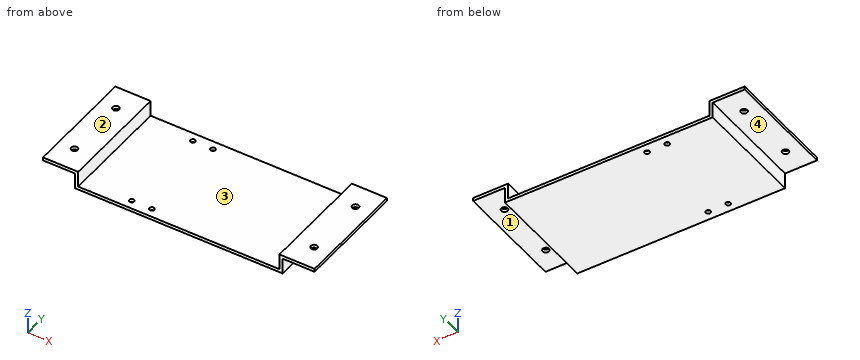
```python
from build123d import *

# Parameters (mm, degrees)
SKETCH1_W           = 126
SKETCH1_H           = 70
BOSS_EXTRUDE1_DEPTH = 2
CUT_EXTRUDE1_REACH  = 4
SKETCH2_R           = 1.5
BOSS_EXTRUDE2_DEPTH = 70
CUT_EXTRUDE2_REACH  = 4
SKETCH4_R           = 2


with BuildPart() as part:
    # Sketch1 → Boss-Extrude1 (new body)
    with BuildSketch(Plane.XY):
        Rectangle(SKETCH1_W, SKETCH1_H)
    extrude(amount=BOSS_EXTRUDE1_DEPTH)

    # Sketch2 → Cut-Extrude1 (cut, up to next)
    with BuildSketch(Plane.XY.offset(2), mode=Mode.PRIVATE) as cut_extrude1_sk1:
        with Locations((-20.4, 29.5)):
            Circle(SKETCH2_R)
    cut_extrude1_tool1 = extrude(cut_extrude1_sk1.sketch, amount=-CUT_EXTRUDE1_REACH, mode=Mode.PRIVATE) & part.part
    add(cut_extrude1_tool1.solids().sort_by_distance((-20.4, 29.5, 2))[0], mode=Mode.SUBTRACT)
    # Sketch2 → Cut-Extrude1 (cut, up to next)
    with BuildSketch(Plane.XY.offset(2), mode=Mode.PRIVATE) as cut_extrude1_sk2:
        with Locations((-33, 29.5)):
            Circle(SKETCH2_R)
    cut_extrude1_tool2 = extrude(cut_extrude1_sk2.sketch, amount=-CUT_EXTRUDE1_REACH, mode=Mode.PRIVATE) & part.part
    add(cut_extrude1_tool2.solids().sort_by_distance((-33, 29.5, 2))[0], mode=Mode.SUBTRACT)
    # Sketch2 → Cut-Extrude1 (cut, up to next)
    with BuildSketch(Plane.XY.offset(2), mode=Mode.PRIVATE) as cut_extrude1_sk3:
        with Locations((-20.4, -29.5)):
            Circle(SKETCH2_R)
    cut_extrude1_tool3 = extrude(cut_extrude1_sk3.sketch, amount=-CUT_EXTRUDE1_REACH, mode=Mode.PRIVATE) & part.part
    add(cut_extrude1_tool3.solids().sort_by_distance((-20.4, -29.5, 2))[0], mode=Mode.SUBTRACT)
    # Sketch2 → Cut-Extrude1 (cut, up to next)
    with BuildSketch(Plane.XY.offset(2), mode=Mode.PRIVATE) as cut_extrude1_sk4:
        with Locations((-33, -29.5)):
            Circle(SKETCH2_R)
    cut_extrude1_tool4 = extrude(cut_extrude1_sk4.sketch, amount=-CUT_EXTRUDE1_REACH, mode=Mode.PRIVATE) & part.part
    add(cut_extrude1_tool4.solids().sort_by_distance((-33, -29.5, 2))[0], mode=Mode.SUBTRACT)

    # Sketch3 → Boss-Extrude2 (add)
    with BuildSketch(Plane(origin=(0, 35, 0), x_dir=(1, 0, 0), z_dir=(0, 1, 0))):
        Polygon((-63, 0), (-63, -12), (-85, -12), (-85, -10), (-65, -10), (-65, 0), align=None)
    boss_extrude2 = extrude(amount=-BOSS_EXTRUDE2_DEPTH)

    # Mirror1: Boss-Extrude2 across plane
    add(boss_extrude2.mirror(Plane(origin=(0, 0, 0), x_dir=(0, 0, 1), z_dir=(1, 0, 0))))

    # Sketch4 → Cut-Extrude2 (cut, up to next)
    with BuildSketch(Plane(origin=(0, 0, 10), x_dir=(-1, 0, 0), z_dir=(0, 0, -1)), mode=Mode.PRIVATE) as cut_extrude2_sk1:
        with Locations((-75, 20)):
            Circle(SKETCH4_R)
    cut_extrude2_tool1 = extrude(cut_extrude2_sk1.sketch, amount=-CUT_EXTRUDE2_REACH, mode=Mode.PRIVATE) & part.part
    add(cut_extrude2_tool1.solids().sort_by_distance((75, 20, 10))[0], mode=Mode.SUBTRACT)
    # Sketch4 → Cut-Extrude2 (cut, up to next)
    with BuildSketch(Plane(origin=(0, 0, 10), x_dir=(-1, 0, 0), z_dir=(0, 0, -1)), mode=Mode.PRIVATE) as cut_extrude2_sk2:
        with Locations((-75, -20)):
            Circle(SKETCH4_R)
    cut_extrude2_tool2 = extrude(cut_extrude2_sk2.sketch, amount=-CUT_EXTRUDE2_REACH, mode=Mode.PRIVATE) & part.part
    add(cut_extrude2_tool2.solids().sort_by_distance((75, -20, 10))[0], mode=Mode.SUBTRACT)
    # Sketch4 → Cut-Extrude2 (cut, up to next)
    with BuildSketch(Plane(origin=(0, 0, 10), x_dir=(-1, 0, 0), z_dir=(0, 0, -1)), mode=Mode.PRIVATE) as cut_extrude2_sk3:
        with Locations((75, 20)):
            Circle(SKETCH4_R)
    cut_extrude2_tool3 = extrude(cut_extrude2_sk3.sketch, amount=-CUT_EXTRUDE2_REACH, mode=Mode.PRIVATE) & part.part
    add(cut_extrude2_tool3.solids().sort_by_distance((-75, 20, 10))[0], mode=Mode.SUBTRACT)
    # Sketch4 → Cut-Extrude2 (cut, up to next)
    with BuildSketch(Plane(origin=(0, 0, 10), x_dir=(-1, 0, 0), z_dir=(0, 0, -1)), mode=Mode.PRIVATE) as cut_extrude2_sk4:
        with Locations((75, -20)):
            Circle(SKETCH4_R)
    cut_extrude2_tool4 = extrude(cut_extrude2_sk4.sketch, amount=-CUT_EXTRUDE2_REACH, mode=Mode.PRIVATE) & part.part
    add(cut_extrude2_tool4.solids().sort_by_distance((-75, -20, 10))[0], mode=Mode.SUBTRACT)


solid = part.part
```
Model file for the job. Use its own axes, mm. Face numbers are marked on the shaded views. A direction names the side the tool comes from. Coordinates: 2 decimals unless noted, no trailing zeros. Write each loop counter-clockwise with the first axis right and the second up, starting at its lowest first coordinate (ties: lowest second). Pieces come first, ordered by that corner, then holes. Notation, with made-up numbers: (88.5, 82) - (140.5, 82) arc R22 ccw to (140.5, 104) - close; hole circle Ø2 at (-35.75, 37). An arc over 180 degrees is marked (long way). One line per item, written item: value. Start each with the question number.
1. Tool access for the marked faces 1 and 2: list every direction of +Z, -Z, +X, -X, +Y, -Y with a clear straight run to the whole face (end or side of a thin tool).
2. Mould opens along X. For the marked faces 3 and 4 say: released by +X, released by -X, zero draft, split by the parting line, or undercut.
3. Flat gauge pins, fed straight in: pin 1 (3 mm diameter, centred on x = -53.5, y = -18, fed in from +Z); pin 2 (6.5 mm diameter, centred on x = 75, y = -20, fed in from -Z); pin 3 (5 mm diameter, centred on y = 3, z = 6, fed in from -X). Where does each tip first touch, or does it go through?
4. Slice it at C-C (x = -33). Write the cut outline in (y, z).
5. Slice it at A-A (y = 20). Write the cut outline in (x, z), plus the area to 3 significant figures.
6. Slice it at B-B (z = 4). Write the cut outline in (x, y).
7. Slice it at D-D (y = -15). Write the cut outline in (x, z), plus the area to 3 significant figures.
8. Probe line 1 (Y direction, x = 75, z = 11.6); line 2 (Y direction, x = -20.4, z = 0.45); line 3 (X direction, y = 4.5, z = 2.75). List the from-to ranges inside material, lowest first. Write a range as from..to.
Answers below:
1. face 1: -Z, +X, +Y, -Y
1. face 2: +Z, +X, -X, +Y, -Y
2. face 3: undercut
2. face 4: zero draft
3. pin 1: stops at z = 2
3. pin 2: stops at z = 10
3. pin 3: stops at x = -65
4. outline: (-35, 0) - (-31, 0) - (-31, 2) - (-35, 2) - close; (-28, 0) - (28, 0) - (28, 2) - (-28, 2) - close; (31, 0) - (35, 0) - (35, 2) - (31, 2) - close
5. outline: (-85, 10) - (-77, 10) - (-77, 12) - (-85, 12) - close; (-73, 10) - (-65, 10) - (-65, 0) - (65, 0) - (65, 10) - (73, 10) - (73, 12) - (63, 12) - (63, 2) - (-63, 2) - (-63, 12) - (-73, 12) - close; (77, 10) - (85, 10) - (85, 12) - (77, 12) - close
5. area: 364 mm^2
6. outline: (-65, -35) - (-63, -35) - (-63, 35) - (-65, 35) - close; (63, -35) - (65, -35) - (65, 35) - (63, 35) - close
7. outline: (-85, 10) - (-65, 10) - (-65, 0) - (65, 0) - (65, 10) - (85, 10) - (85, 12) - (63, 12) - (63, 2) - (-63, 2) - (-63, 12) - (-85, 12) - close
7. area: 380 mm^2
8. line 1: y = -35..-22, -18..18, 22..35
8. line 2: y = -35..-31, -28..28, 31..35
8. line 3: x = -65..-63, 63..65
